from build123d import *

# Parameters (mm, degrees)
SALIENTE_EXTRUIR1_DEPTH = 15
CHAFL_N1_SIZE           = 3
CORTAR_EXTRUIR1_START   = -10
CROQUIS3_W              = 16
CROQUIS3_H              = 16
CORTAR_EXTRUIR1_DEPTH   = 31
CHAFL_N2_SIZE           = 3
CROQUIS4_R              = 3.2
CORTAR_EXTRUIR2_DEPTH   = 14
REDONDEO1_R             = 3


with BuildPart() as part:
    # Croquis1 → Saliente-Extruir1 (new body, symmetric)
    with BuildSketch(Plane.XY):
        Polygon((-30, 0), (-30, 10), (0, 40), (0, 10), (15, 10), (15, 0), (0, 0), (-10.471019058, 0), (-11, -3), (-19, -3), (-19.528980942, 0), align=None)
    extrude(amount=SALIENTE_EXTRUIR1_DEPTH, both=True)

    # Chaflán1
    chafl_n1_edges = [part.edges().sort_by_distance(p)[0] for p in [
        (-30, 5, -15),
        (15, 5, 15),
        (15, 5, -15),
        (-30, 5, 15),
    ]]
    chamfer(chafl_n1_edges, length=CHAFL_N1_SIZE)

    # Croquis3 → Cortar-Extruir1 (cut, through all)
    with BuildSketch(Plane.XZ.offset(CORTAR_EXTRUIR1_START)):
        with Locations((-15, 0)):
            Rectangle(CROQUIS3_W, CROQUIS3_H)
    extrude(amount=-CORTAR_EXTRUIR1_DEPTH, mode=Mode.SUBTRACT)

    # Chaflán2
    chafl_n2_edges = [part.edges().sort_by_distance(p)[0] for p in [
        (-23, 13.5, -8),
        (-23, 13.5, 8),
        (-7, 21.5, 8),
        (-7, 21.5, -8),
    ]]
    chamfer(chafl_n2_edges, length=CHAFL_N2_SIZE)

    # Croquis4 → Cortar-Extruir2 (cut, through all)
    with BuildSketch(Plane(origin=(0, 10, 0), x_dir=(1, 0, 0), z_dir=(0, 1, 0))):
        with Locations((-15, 0)):
            Circle(CROQUIS4_R)
    extrude(amount=-CORTAR_EXTRUIR2_DEPTH, mode=Mode.SUBTRACT)

    # Redondeo1
    redondeo1_edges = [part.edges().sort_by_distance(p)[0] for p in [
        (0, 40, 0),
    ]]
    fillet(redondeo1_edges, radius=REDONDEO1_R)


solid = part.part
Could you check a few things on this model? Use its own coordinates, in mm. A direction names the side the tool comes from. Give positions to 0.01 mm unless a question says otherwise; leave off trailing zeros. Order: outer loops, then holes, each group sorted by start corner. A loop starts at its lowest first (then second) coordinate and runs counter-clockwise, first axis right, second up.
1. Suppose I cut it at A-A (y = 3.5). Write out the boundary of the cut face in (x, z), plus the area to 3 significant figures.
Answers below:
outline: (-30, -12) - (-27, -15) - (12, -15) - (15, -12) - (15, 12) - (12, 15) - (-27, 15) - (-30, 12) - close; hole circle Ø6.4 at (-15, 0)
area: 1,300 mm2
2. Which directions (+Z, -Z, +X, -X, +Y, -Y) give clear straight access to the entire face, cutting with the end or side of a thin tool? Please do faces 5 (the flat face through (0, 22, 0)), 6 (the flat face through (-15, 18, -8)), 7 (the flat face through (-25, 0, 0)).
Answers below:
face 5: +Z, -Z, +X, +Y
face 6: +Y
face 7: +Z, -Z, -X, -Y
3. Suppose I cut it at C-C (x = -15). Write out the boundary of the cut face in (y, z), plus the area to 3 significant figures.
Answers below:
outline: (-3, -15) - (25, -15) - (25, -8) - (10, -8) - (10, -3.2) - (-3, -3.2) - close; (-3, 3.2) - (10, 3.2) - (10, 8) - (25, 8) - (25, 15) - (-3, 15) - close
area: 517 mm2
4. I need wall thicknesses on L1, parallel to X at y = 3.25, z = 0; L2, parallel to Z at x = -15, y = 2.5; L3, parallel to Z at x = -19.5, y = 14. Which ranges of each line are inside material? Lowest first, please.
Answers below:
L1: x = -30 to -18.2, -11.8 to 15
L2: z = -15 to -3.2, 3.2 to 15
L3: z = -15 to -8, 8 to 15
5. Suppose I cut it at D-D (z = -4). Write out the boundary of the cut face in (x, y).
Answers below:
outline: (-30, 0) - (-19.53, 0) - (-19, -3) - (-11, -3) - (-10.47, 0) - (15, 0) - (15, 10) - (0, 10) - (0, 32.76) arc R3 ccw to (-5.12, 34.88) - (-7, 33) - (-7, 10) - (-23, 10) - (-23, 17) - (-30, 10) - close
6. Suppose I cut it at B-B (z = 0). Write out the boundary of the cut face in (x, y), plus the area to 3 significant figures.
Answers below:
outline: (-30, 0) - (-19.53, 0) - (-19, -3) - (-18.2, -3) - (-18.2, 10) - (-23, 10) - (-23, 17) - (-30, 10) - close; (-11.8, -3) - (-11, -3) - (-10.47, 0) - (15, 0) - (15, 10) - (0, 10) - (0, 32.76) arc R3 ccw to (-5.12, 34.88) - (-7, 33) - (-7, 10) - (-11.8, 10) - close
area: 591 mm2
7. For pin 1 (2 mm diameter, centred on x = 2.5, z = -5, fed in from -Y); pin 2 (17.5 mm diameter, centred on x = -13.5, z = -1, fed in from +Y); pin 3 (1.5 mm diameter, centred on y = 25.5, z = -8.5, fed in from -X), each with a flat end and sliding along its axis, tell me the tip position at first contact or that it passes through.
Answers below:
pin 1: stops at y = 0
pin 2: stops at y = 35.19
pin 3: stops at x = -15.25
8. Thinking about a two-plate mould opening in Z: for faces 1 (the flat face through (-28, 6, 14)), 2 (the flat face through (-22, 14, -6)), 3 (the flat face through (-7, 12, -15)), 4 (the flat face through (-15, -3, 4)), which applies, +Z half, -Z half, draft (parallel to the pull), parting line (faces both ways), or undercut?
Answers below:
face 1: +Z half
face 2: undercut
face 3: -Z half
face 4: draft
